from build123d import *

# Parameters (mm, degrees)
SKETCH1_W               = 120
SKETCH1_H               = 80
BOSS_EXTRUDE1_DEPTH     = 3
SKETCH2_R               = 4
CUT_EXTRUDE1_DEPTH      = 2
MIRROR2_COPY_1_SKETCH_R = 4
MIRROR2_COPY_1_DEPTH    = 2
FILLET2_R               = 3


with BuildPart() as part:
    # Sketch1 → Boss-Extrude1 (new body)
    with BuildSketch(Plane(origin=(0, 0, 0), x_dir=(1, 0, 0), z_dir=(0, 1, 0))):
        with Locations((60, 40)):
            Rectangle(SKETCH1_W, SKETCH1_H)
    extrude(amount=BOSS_EXTRUDE1_DEPTH)

    # Sketch2 → Cut-Extrude1 (cut)
    with BuildSketch(Plane(origin=(0, 3, 0), x_dir=(1, 0, 0), z_dir=(0, 1, 0))):
        with Locations(Location((5, 75, 0), (0, 0, 270))):
            Circle(SKETCH2_R)
    cut_extrude1 = extrude(amount=-CUT_EXTRUDE1_DEPTH, mode=Mode.SUBTRACT)

    # Mirror1: Cut-Extrude1 across plane
    add(cut_extrude1.mirror(Plane(origin=(0, 0, -40), x_dir=(1, 0, 0), z_dir=(0, 0, -1))), mode=Mode.SUBTRACT)

    # Mirror2: Cut-Extrude1 across plane
    add(cut_extrude1.mirror(Plane.ZY.offset(-60)), mode=Mode.SUBTRACT)

    # Mirror2 copy 1 sketch → Mirror2 copy 1 (cut)
    with BuildSketch(Plane(origin=(120, 3, -80), x_dir=(-1, 0, 0), z_dir=(0, 1, 0))):
        with Locations(Location((5, 75, 0), (0, 0, 270))):
            Circle(MIRROR2_COPY_1_SKETCH_R)
    extrude(amount=-MIRROR2_COPY_1_DEPTH, mode=Mode.SUBTRACT)

    # Fillet2
    fillet2_edges = [part.edges().sort_by_distance(p)[0] for p in [
        (0, 1.5, -80),
        (120, 1.5, -80),
        (120, 1.5, 0),
        (0, 1.5, 0),
    ]]
    fillet(fillet2_edges, radius=FILLET2_R)


solid = part.part
CAD build for the part. Positions are in the model's coordinates, mm. A direction names the side the tool comes from. Round coordinates to 2 decimals unless told otherwise and drop trailing zeros. Write each loop counter-clockwise with the first axis right and the second up, starting at its lowest first coordinate (ties: lowest second). Pieces come first, ordered by that corner, then holes. Notation, with made-up numbers: M 31.5,-17 L 39.5,-17 A25 ccw 39.5,7 Z; hole C -21,42.5 d8. An arc over 180 degrees is marked long. Use a Markdown table: item, result. Add a question column.
1. Slice it at A-A on y = 1.6. Give the cut face in (x, z).
2. Slice it at B-B on z = -75. Give the cut face in (x, y).
3. Drill centre lines: probe 1 along Z at (x, y) = (115, 1.75); probe 2 along X at (y, z) = (2.2, -5). Where is each one in solid material? Low to high.
4. Slice it at C-C on x = 5. Give the cut face in (y, z), then the cut area to 3 significant figures.
5. 3-axis set-ups, long thin cutter, end or side, ignore diameter. For faces 1 (the face through (115, 1, -75)), 2 (the face through (119.1, 1.52, -0.86)): which of +Z, -Z, +X, -X, +Y, -Y reach the whole face in a straight line?
6. Flat gauge pin, fed straight in: P1, Ø2.5, axis at x = 117, z = -75.5, coming from the +Y side. Where does the tip first touch, or does it go through?
7. Pull direction X, two halves, no side cores. Call faces 3 (the face through (5, 2, -79)), 4 (the face through (0.86, 1.52, -79.1)), 5 (the face through (59, 1, -80)): released by +X, released by -X, zero draft, split by the parting line, or undercut.
Reply:
| question | item | result |
|---|---|---|
| 1 | outline | M 0,-77 A3 ccw 3,-80 L 117,-80 A3 ccw 120,-77 L 120,-3 A3 ccw 117,0 L 3,0 A3 ccw 0,-3 Z; hole C 5,-75 d8; hole C 5,-5 d8; hole C 115,-75 d8; hole C 115,-5 d8 |
| 2 | outline | M 0,0 L 120,0 L 120,3 L 119,3 L 119,1 L 111,1 L 111,3 L 9,3 L 9,1 L 1,1 L 1,3 L 0,3 Z |
| 3 | probe 1 | z = -80 to -79, -71 to -9, -1 to 0 |
| 3 | probe 2 | x = 0 to 1, 9 to 111, 119 to 120 |
| 4 | outline | M 0,-80 L 3,-80 L 3,-79 L 1,-79 L 1,-71 L 3,-71 L 3,-9 L 1,-9 L 1,-1 L 3,-1 L 3,0 L 0,0 Z |
| 4 | area | 208 mm^2 |
| 5 | face 1 | +Y |
| 5 | face 2 | +Z, +X, +Y, -Y |
| 6 | P1 | stops at y = 1 |
| 7 | face 3 | undercut |
| 7 | face 4 | released by -X |
| 7 | face 5 | zero draft |
